Check sheet for the drawn part. Datum: minimum x, y, z corner. Units: mm. Round coordinates to 2 decimals unless told otherwise and drop trailing zeros. Write each loop counter-clockwise with the first axis right and the second up, starting at its lowest first coordinate (ties: lowest second). Pieces come first, ordered by that corner, then holes. Notation, with made-up numbers: M 28,-2 L 73,-2 A16 cw 73,3 Z; hole C 11.5,0 d8. An arc over 180 degrees is marked long. Use a Markdown table: item, result.
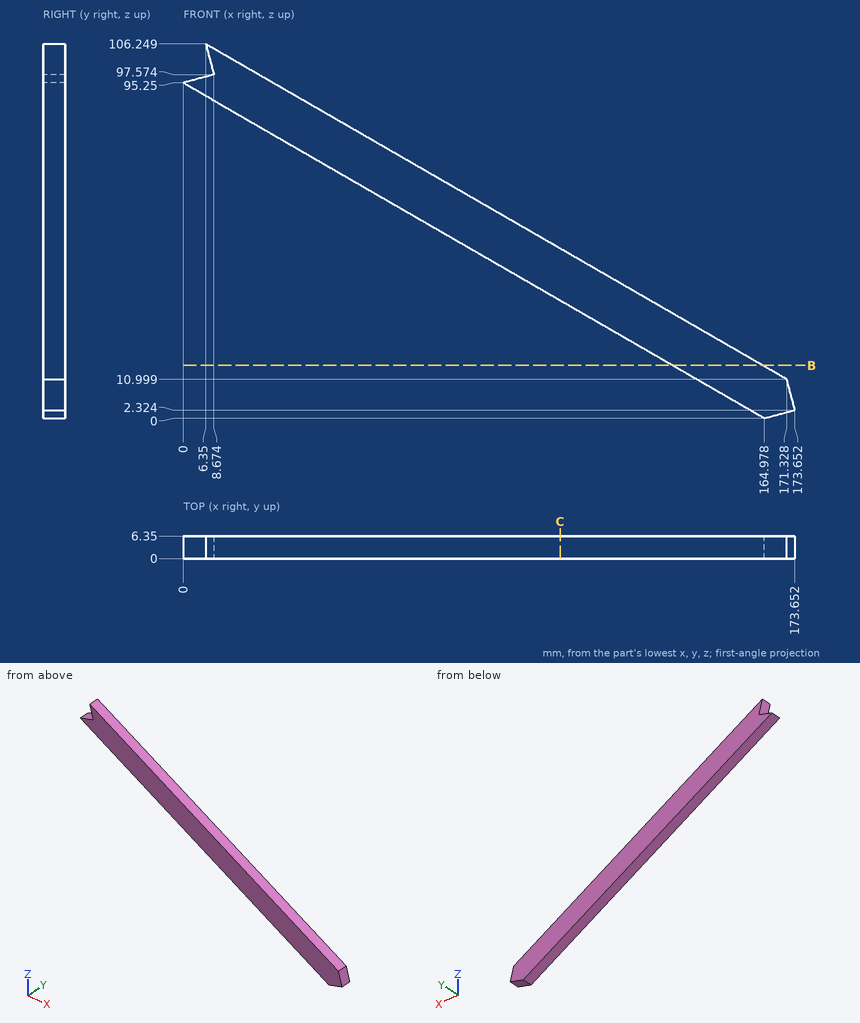
Item 1: Cross-section at C-C, the plane x = 107. Record the cut outline in (y, z).
Outcome:
| item | result |
|---|---|
| outline | M 0,33.47 L 6.35,33.47 L 6.35,48.14 L 0,48.14 Z |
Item 2: Go/stop test with flat-tipped pins: pin 1 (3 mm diameter, centred on y = 3.5, z = 50.5, fed in from -X); pin 2 (2 mm diameter, centred on x = 101.5, y = 1.5, fed in from -Z); pin 3 (1.5 mm diameter, centred on y = 2.5, z = 34, fed in from +X) (1 decimal). Record where each tip stops, or that it passes through.
Outcome:
| item | result |
|---|---|
| pin 1 | stops at x = 74.91 |
| pin 2 | stops at z = 36.07 |
| pin 3 | stops at x = 132.8 |
Item 3: Cross-section at B-B, the plane z = 15. Record the cut outline in (x, y).
Outcome:
| item | result |
|---|---|
| outline | M 139,0 L 164.4,0 L 164.4,6.35 L 139,6.35 Z |
Item 4: Material ranges on line 1 along Z through (x, y) = (36, 5.5) (1 decimal); line 2 along X through (y, z) = (3.5, 17) (1 decimal); line 3 along Z through (x, y) = (129, 0.75) (1 decimal), recorded low to high. Write a range as from..to.
Outcome:
| item | result |
|---|---|
| line 1 | z = 74.5..89.1 |
| line 2 | x = 135.5..160.9 |
| line 3 | z = 20.8..35.4 |
